Autodesk Inventor part; units mm, degrees
ref_plane "YZ Plane" through (0, 0, 0) normal (1, 0, 0) x (0, 1, 0)
ref_plane "XZ Plane" through (0, 0, 0) normal (0, 1, 0) x (-1, 0, 0)
ref_plane "XY Plane" through (0, 0, 0) normal (0, 0, 1) x (1, 0, 0)
sketch "Sketch1" plane through (0, 0, 0) normal (0, 1, 0) x (-1, 0, 0)
  line L0 (-7.5, -4.5) -> (7.5, -4.5)
  line L1 (7.5, -4.5) -> (7.5, 4.5)
  line L2 (7.5, 4.5) -> (-7.5, 4.5)
  line L3 (-7.5, 4.5) -> (-7.5, -4.5)
  line L4 (-7.5, -4.5) -> (7.5, 4.5) construction
  line L5 (7.5, -4.5) -> (-7.5, 4.5) construction
  circle A0 centre (7.5, 0) radius 1.5
  circle A1 centre (7.5, 0) radius 4.5
  point P0 (0, 0)
  dimension "d0" = 15
  dimension "d1" = 3
  dimension "d2" = 9
  dimension "d3" = 9
extrude "Extrusion1" add sketch "Sketch1" along normal blind 3 contours L3 L2 A1 L0 | A1 L1 A0 | L1 A0 A1 | A0 L1 picked at (7.0325, 0.1773)
sketch "Sketch2" plane through (0, 3, 0) normal (0, 1, 0) x (1, 0, 0)
  line L0 (-7.5, -1.5) -> (-7.5, 1.5)
  circle A0 centre (-7.5, 0) radius 1.5
  point P0 (0, 0)
  dimension "d6" = 3
extrude "Extrusion2" cut sketch "Sketch2" against normal blind 3
sketch "Sketch3" plane through (0, 3, 0) normal (0, 1, 0) x (1, 0, 0)
  line L0 (7.5, 4.5) -> (-7.5, 4.5)
  line L1 (4.5, 4.5) -> (-0.5, 4.5)
  line L2 (-0.5, 4.5) -> (-0.5, 7.5)
  line L3 (-0.5, 7.5) -> (4.5, 7.5)
  line L4 (4.5, 7.5) -> (4.5, 4.5)
  line L5 (7.5, -4.5) -> (7.5, 4.5)
  point P0 (0, 0)
  dimension "d9" = 5
  dimension "d10" = 3
  dimension "d11" = 3
extrude "Extrusion3" add sketch "Sketch3" against normal blind 3
fillet "Fillet1" radius 9 1 edges at (7.5, 1.5, 4.5)
properties part number "Bottom battery holder"
Input: part model. Units: mm. Frame: model coordinates. A direction names the side the tool comes from. Give positions to 0.01 mm unless a question says otherwise; leave off trailing zeros. Order: outer loops, then holes, each group sorted by start corner. A loop starts at its lowest first (then second) coordinate and runs counter-clockwise, first axis right, second up.
Q1. Contact query for flat-ended pins moving along their axis: pin 1 Ø3 at (x, z) = (-6.5, -2) entering from -Y; pin 2 Ø0.9 at (x, y) = (6.5, 1) entering from -Z; pin 3 Ø2.5 at (x, z) = (-7.5, 0) entering from +Y; pin 4 Ø1.5 at (y, z) = (2.5, 1.5) entering from -X. Output: stop coordinate, or through.
Checked values:
pin 1: stops at y = 0
pin 2: stops at z = -4.5
pin 3: passes through
pin 4: stops at x = -11.94
Q2. Section D-D on x = -3. Output: boundary loops of the cut face in (y, z), and give its area (3 significant figures).
Checked values:
outline: (0, -4.5) - (3, -4.5) - (3, 4.5) - (0, 4.5) - close
area: 27.0 mm2
Q3. Set-up query: faces 1 (the flat face through (4.5, 2, -6)), 2 (the flat face through (-0.5, 2, -6)), 3 (the cylindrical face through (-12, 1, 0)). Return all of +Z, -Z, +X, -X, +Y, -Y with unobstructed straight access to the full face (end or side cutting, diameter ignored); none if empty.
Checked values:
face 1: -Z, +X, +Y, -Y
face 2: -Z, -X, +Y, -Y
face 3: -X, +Y, -Y
Q4. Ray query, probe 1 along Z at (x, y) = (-7.5, 2); probe 2 along Z at (x, y) = (-1.25, 1.55); probe 3 along X at (y, z) = (1.05, 0). Return the intervals inside material, ascending.
Checked values:
probe 1: z = -4.5 to -1.5, 1.5 to 4.5
probe 2: z = -4.5 to 4.5
probe 3: x = -12 to -9, -6 to 6.29
Q5. Draft query along Z for faces 4 (the cylindrical face through (-9, 1, 0)), 5 (the cylindrical face through (4.794, 1.521, 1.934)), 6 (the flat face through (-2, 3, -1)). Return one class per face: +Z half, -Z half, draft (parallel to the pull), parting line (faces both ways), or undercut.
Checked values:
face 4: undercut
face 5: +Z half
face 6: draft
Q6. Section C-C on x = -6.5. Output: boundary loops of the cut face in (y, z), and give its area (3 significant figures).
Checked values:
outline: (0, -4.5) - (3, -4.5) - (3, -1.12) - (0, -1.12) - close; (0, 1.12) - (3, 1.12) - (3, 4.5) - (0, 4.5) - close
area: 20.3 mm2
Q7. Section A-A on z = 0. Output: boundary loops of the cut face in (x, y).
Checked values:
outline: (-12, 0) - (-9, 0) - (-9, 3) - (-12, 3) - close; (-6, 0) - (6.29, 0) - (6.29, 3) - (-6, 3) - close
